Build history of the part. All positions in model axes, mm. Face numbers are marked on the shaded views. A direction names the side the tool comes from. Coordinates: 2 decimals unless noted, no trailing zeros. Order: outer loops, then holes, each group sorted by start corner. A loop starts at its lowest first (then second) coordinate and runs counter-clockwise, first axis right, second up. Notation, with made-up numbers: (-8.5, 45) -> (31.5, 45) arc R34 ccw to (31.5, 76) -> close; hole circle Ø11 at (88, 61). An arc over 180 degrees is marked (long way). Write each question's results on one line, items separated by ' | '.
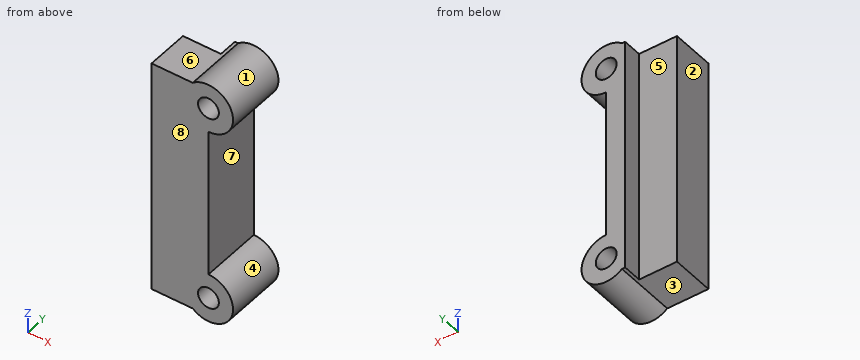
Autodesk Inventor part; units mm, degrees
ref_plane "YZ Plane" through (0, 0, 0) normal (1, 0, 0) x (0, 1, 0)
ref_plane "XZ Plane" through (0, 0, 0) normal (0, 1, 0) x (-1, 0, 0)
ref_plane "XY Plane" through (0, 0, 0) normal (0, 0, 1) x (1, 0, 0)
sketch "Sketch1" plane through (0, 0, 0) normal (0, 1, 0) x (-1, 0, 0)
  line L0 (4.5194, 15.534) -> (-1.4806, 15.534)
  line L1 (-1.4806, 15.534) -> (-1.4806, -9.466)
  line L2 (-1.4806, -9.466) -> (4.5194, -9.466)
  line L3 (4.5194, -9.466) -> (4.5194, 15.534)
  point P0 (0, 0)
  dimension "d0" = 25
  dimension "d1" = 6
extrude "Extrusion1" add sketch "Sketch1" along normal blind 4.5
sketch "Sketch2" plane through (0, 4.5, 0) normal (0, 1, 0) x (1, 0, 0)
  line L0 (1.4806, -15.534) -> (1.4806, 9.466)
  line L1 (-4.5194, -15.534) -> (1.4806, -15.534)
  line L2 (-0.1807, 9.466) -> (-0.5194, 9.466)
  line L3 (-0.5194, 9.466) -> (-0.5194, -15.534)
  line L4 (-0.5194, -15.534) -> (-0.1807, -15.534)
  circle A0 centre (1.4806, 7.466) radius 1.1
  circle A1 centre (1.4806, -13.534) radius 1.1
  arc A2 (-0.1807, -15.534) -> (1.4806, -10.934) centre (1.4806, -13.534) ccw
  arc A3 (1.4806, 4.866) -> (-0.1807, 9.466) centre (1.4806, 7.466) ccw
  line L5 (1.4806, -10.934) -> (1.4806, 4.866)
  point P0 (0, 0)
  point P1 (1.4806, 10.066)
  point P2 (1.4806, -16.134)
  dimension "d4" = 2
  dimension "d5" = 2.2
  dimension "d6" = 0
  dimension "d8" = 2
  dimension "d9" = 2.2
  dimension "d10" = 0
  dimension "d11" = 2
  dimension "d17" = 1.5
  dimension "d18" = 1.5
extrude "Extrusion3" add sketch "Sketch2" along normal blind 2 and the other way blind 4.5 contours L0 A1 L1 L3 L2 A3 | A2 L1 L0 A1
extrude "Extrusion4" cut sketch "Sketch2" along normal through all both and the other way through all contours A0 L0 | L0 A0 | A1 L0 | L0 A1
properties part number "rectSotto"
Item 1: Slice it at A-A, the plane z = 8.25. List the corners of the cut face in (x, y).
Answer:
outline: (-4.52, 0) -> (1.48, 0) -> (1.48, 6.5) -> (-0.52, 6.5) -> (-0.52, 4.5) -> (-4.52, 4.5) -> close
Item 2: Drill centre lines: line 1 (Z direction, x = 0.5, y = 0.5); line 2 (X direction, y = 2.25, z = -4); line 3 (Y direction, x = -3.5, z = 12.5). Where is each one in solid material? Low to high. Write a range as from..to.
Answer:
line 1: z = -9.87..-7.96, -6.97..13.04, 14.03..15.94 | line 2: x = -4.52..1.48 | line 3: y = 0..4.5
Item 3: Slice it at D-D, the plane z = -8. List the corners of the cut face in (x, y).
Answer:
outline: (-4.52, 0) -> (0.52, 0) -> (0.52, 6.5) -> (-0.52, 6.5) -> (-0.52, 4.5) -> (-4.52, 4.5) -> close; (2.44, 0) -> (4.03, 0) -> (4.03, 6.5) -> (2.44, 6.5) -> close
Item 4: Pull direction Z, two halves, no side cores. Call the marked faces 1, 2, 3 and 4: released by +Z, released by -Z, zero draft, split by the parting line, or undercut.
Answer:
face 1: undercut | face 2: zero draft | face 3: released by -Z | face 4: undercut
Item 5: Tool access for the marked faces 5, 6, 7 and 8: list every direction of +Z, -Z, +X, -X, +Y, -Y with a clear straight run to the whole face (end or side of a thin tool).
Answer:
face 5: +Z, -Z, -X, +Y | face 6: +Z, -X, +Y, -Y | face 7: +X, +Y, -Y | face 8: +Z, -Z, +X, -X, -Y
Item 6: Slice it at C-C, the plane x = 1.75. List the corners of the cut face in (y, z), and give its area (3 significant figures).
Answer:
outline: (0, -10.05) -> (6.5, -10.05) -> (6.5, -8.53) -> (0, -8.53) -> close; (0, -6.4) -> (6.5, -6.4) -> (6.5, -4.88) -> (0, -4.88) -> close; (0, 10.95) -> (6.5, 10.95) -> (6.5, 12.47) -> (0, 12.47) -> close; (0, 14.6) -> (6.5, 14.6) -> (6.5, 16.12) -> (0, 16.12) -> close | area: 39.5 mm^2
Item 7: Pin check, flat tips, straight feed: pin 1 (2 mm diameter, centred on x = 1.48, z = -7.47, fed in from +Y); pin 2 (3 mm diameter, centred on x = -2, y = 4.5, fed in from -Z); pin 3 (3 mm diameter, centred on x = -3, z = 1, fed in from +Y); pin 4 (2 mm diameter, centred on x = -2.5, y = 1.5, fed in from +Z). Stop position of each tip, or through.
Answer:
pin 1: passes through | pin 2: stops at z = -9.47 | pin 3: stops at y = 4.5 | pin 4: stops at z = 15.53
Item 8: Slice it at B-B, the plane y = 6. List the corners of the cut face in (x, z).
Answer:
outline: (-0.52, -9.47) -> (-0.18, -9.47) arc R2.6 ccw (long way) to (1.48, -4.87) -> (1.48, 10.93) arc R2.6 ccw (long way) to (-0.18, 15.53) -> (-0.52, 15.53) -> close; hole circle Ø2.2 at (1.48, -7.47); hole circle Ø2.2 at (1.48, 13.53)
